Model file for the job. Use its own axes, mm. A direction names the side the tool comes from. Coordinates: 2 decimals unless noted, no trailing zeros. Order: outer loops, then holes, each group sorted by start corner. A loop starts at its lowest first (then second) coordinate and runs counter-clockwise, first axis right, second up. Notation, with made-up numbers: (2, -6.5) -> (55, -6.5) arc R24 ccw to (55, 25.5) -> close; hole circle Ø1 at (79.25, 40.5). An arc over 180 degrees is marked (long way). Write item = value, one per line. Start each with the question number.
Q1. Cut at A-A, the plane x = 0. List the corners of the cut face in (y, z), plus the area to 3 significant figures.
Q2. Cut at D-D, the plane y = -12.5. List the corners of the cut face in (x, z), plus the area to 3 significant figures.
Q3. Wall check: line 1 (Y direction, x = 0, z = 0.75); line 2 (Y direction, x = 0, z = 5.75); line 3 (X direction, y = 3, z = 0.5). Give the ranges that are in metal, low to high. Write a range as from..to.
Q4. Mould opens along Y. For faces 4 (the face through (6, -6, 9)), 5 (the face through (6.691, -12.864, 9.507)), 6 (the face through (-3.47, 15.62, 4.93)), 7 (the face through (2, 6, 0)) say: +Y half, -Y half, draft (parallel to the pull), parting line (faces both ways), or undercut.
Q5. 3-axis set-ups, long thin cutter, end or side, ignore diameter. For faces 1 (the face through (6.691, 12.864, 0.493)), 2 (the face through (-6, 0, 5)), 3 (the face through (-7.493, 0.33, 9.507)): which of +Z, -Z, +X, -X, +Y, -Y reach the whole face in a straight line?
Q6. Flat gauge pins, fed straight in: pin 1 (3 mm diameter, centred on y = 6, z = 4.5, fed in from +X); pin 2 (1 mm diameter, centred on x = -3.5, y = 11, fed in from -Z); pin 3 (4 mm diameter, centred on x = -3.5, z = 5, fed in from +Y). Where does each tip first touch, or does it go through?
Q7. Cut at C-C, the plane z = 3.25. List the corners of the cut face in (x, y).
Autodesk Inventor part; units mm, degrees
ref_plane "Work Plane1" through (0, 0, 5) normal (0, 0, 1) x (1, 0, 0)
ref_plane "YZ Plane" through (0, 0, 0) normal (1, 0, 0) x (0, 1, 0)
ref_plane "XZ Plane" through (0, 0, 0) normal (0, 1, 0) x (-1, 0, 0)
sketch "Sketch1" plane through (0, 0, 0) normal (0, 0, 1) x (1, 0, 0)
  circle A0 centre (0, 0) radius 6
  circle A1 centre (0, 0) radius 16
  dimension "d0" = 12
  dimension "d1" = 32
extrude "Extrusion1" add sketch "Sketch1" along normal blind 10
sketch "Sketch2" plane through (0, 0, 10) normal (0, 0, 1) x (1, 0, 0)
  circle A0 centre (0, 0) radius 16
  circle A1 centre (0, 0) radius 6
  circle A2 centre (0, 0) radius 7.5
  circle A3 centre (0, 0) radius 14.5
  dimension "d4" = 1.5
  dimension "d5" = 1.5
extrude "Extrusion2" cut sketch "Sketch2" against normal blind 1 contours A3
ref_plane "Work Plane1" through (0, 0, 5) normal (0, 0, 1) x (1, 0, 0)
mirror "Mirror1" about plane through (0, 0, 5) normal (0, 0, 1) of "Extrusion2"
properties part number "6201 Bearing"
Here are the results:
q1.outline = (-16, 0) -> (-14.5, 0) -> (-14.5, 1) -> (-7.5, 1) -> (-7.5, 0) -> (-6, 0) -> (-6, 10) -> (-7.5, 10) -> (-7.5, 9) -> (-14.5, 9) -> (-14.5, 10) -> (-16, 10) -> close; (6, 0) -> (7.5, 0) -> (7.5, 1) -> (14.5, 1) -> (14.5, 0) -> (16, 0) -> (16, 10) -> (14.5, 10) -> (14.5, 9) -> (7.5, 9) -> (7.5, 10) -> (6, 10) -> close
q1.area = 172 mm²
q2.outline = (-9.99, 0) -> (-7.35, 0) -> (-7.35, 1) -> (7.35, 1) -> (7.35, 0) -> (9.99, 0) -> (9.99, 10) -> (7.35, 10) -> (7.35, 9) -> (-7.35, 9) -> (-7.35, 10) -> (-9.99, 10) -> close
q2.area = 170 mm²
q3.line_1 = -16..-14.5, -7.5..-6, 6..7.5, 14.5..16
q3.line_2 = -16..-6, 6..16
q3.line_3 = -15.72..-14.19, -6.87..-5.2, 5.2..6.87, 14.19..15.72
q4.face_4 = undercut
q4.face_5 = undercut
q4.face_6 = parting line
q4.face_7 = draft
q5.face_1 = -Z
q5.face_2 = +Z, -Z
q5.face_3 = +Z
q6.pin_1 = 15.35
q6.pin_2 = 1
q6.pin_3 = 15.93
q7.outline = circle Ø32 at (0, 0); hole circle Ø12 at (0, 0)
